Autodesk Inventor part; units mm, degrees
ref_plane "YZ Plane" through (0, 0, 0) normal (1, 0, 0) x (0, 1, 0)
ref_plane "XZ Plane" through (0, 0, 0) normal (0, 1, 0) x (-1, 0, 0)
ref_plane "XY Plane" through (0, 0, 0) normal (0, 0, 1) x (1, 0, 0)
sketch "Sketch1" plane through (0, 0, 0) normal (0, 0, 1) x (1, 0, 0)
  line L0 (0, 0) -> (0, -500) construction
  line L1 (0, 0) -> (6, 0)
  line L2 (6, 0) -> (6, -60)
  line L3 (6, -60) -> (9.2, -60)
  line L4 (9.2, -60) -> (9.2, -140)
  line L5 (9.2, -140) -> (6, -140)
  line L6 (6, -140) -> (6, -232.5)
  line L7 (0, 0) -> (0, -443)
  line L8 (0, 0) -> (0, 9) construction
  line L9 (4, -443) -> (4, -232.5)
  line L10 (4, -232.5) -> (6, -232.5)
  line L11 (4, -443) -> (0, -443)
  dimension "d1" = 12
  dimension "d2" = 60
  dimension "d3" = 18.4
  dimension "d4" = 80
  dimension "d7" = 8
  dimension "d8" = 210.5
  dimension "d9" = 443
revolve "Revolution1" add sketch "Sketch1" angle 360 about axis through (0, 0, 0) along (0, -1, 0)
sketch "Sketch2" plane through (0, -232.5, 0) normal (0, -1, 0) x (1, 0, 0)
  line L0 (0, 0) -> (0, 10.7217) construction
  line L1 (0, 0) -> (0, -10) construction
  line L2 (0, 0) -> (-12.4689, 0) construction
  line L3 (0, 0) -> (11.6918, 0) construction
  circle A0 centre (0, 0) radius 6 construction
  arc A1 (6, 0) -> (0, 6) centre (0, 0) ccw
  arc A2 (-6, 0) -> (0, -6) centre (0, 0) ccw
  arc A3 (4, 0) -> (0, 4) centre (0, 0) ccw
  arc A4 (-4, 0) -> (0, -4) centre (0, 0) ccw
  line L4 (-4, 0) -> (-6, 0)
  line L5 (0, -4) -> (0, -6)
  line L6 (0, 4) -> (0, 6)
  line L7 (4, 0) -> (6, 0)
  dimension "d10" = 4
  dimension "d11" = 4
extrude "Extrusion1" add sketch "Sketch2" along normal blind 5
sketch "Sketch3" plane through (0, -443, 0) normal (0, -1, 0) x (1, 0, 0)
  point P0 (0, 0)
  point P1 (0, 0)
hole "Hole1" at (0, -443, 0) direction (0, 1, 0) diameter 1.567 depth 6.3 tip angle 118
sketch "Sketch4" plane through (0, -443, 0) normal (0, -1, 0) x (1, 0, 0)
  point P0 (0, 0)
properties part number "Achse"
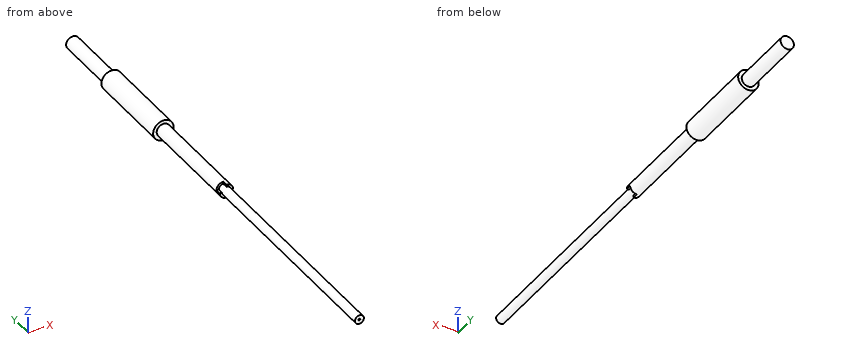
Part model, mm, in its own coordinate system. Coordinates: 2 decimals unless noted, no trailing zeros. Loops run counter-clockwise (first coordinate to the right, second up) from the corner with the lowest first, then second, coordinate; pieces in that order, holes last. Notation, with made-up numbers: (32, 13) - (37, 13) arc R21 ccw to (37, 40) - close; hole circle Ø7 at (18.25, 85.25). An arc over 180 degrees is marked (long way). Write item = value, one per line. Start each with the question number.
Item 1: Flat gauge pins, fed straight in: pin 1 Ø1.6 at (x, y) = (-4.5, -235.5) entering from +Z; pin 2 Ø8 at (y, z) = (-253.5, -7.5) entering from -X; pin 3 Ø1.6 at (y, z) = (-235, 5) entering from -X. Where does each tip first touch, or does it go through?
Item 2: Wall check: L1, parallel to X at y = -438, z = 0; L2, parallel to Y at x = -2.75, z = -6.75. Give the ranges that are in metal, low to high. Write a range as from..to.
Item 3: Cut at B-B, the plane y = -166.5. Give the cut face in (x, z), and give its area (3 significant figures).
Item 4: Cut at A-A, the plane y = -322. Give the cut face in (x, z).
The answers:
q1.pin_1 = 1.52
q1.pin_2 = -1.94
q1.pin_3 = 0
q2.L1 = -4..-0.78, 0.78..4
q2.L2 = -140..-60
q3.outline = circle Ø12 at (0, 0)
q3.area = 113 mm2
q4.outline = circle Ø8 at (0, 0)
